Could you check a few things on this model? Use its own coordinates, in mm. A direction names the side the tool comes from. Give positions to 0.01 mm unless a question says otherwise; leave off trailing zeros. Order: outer loops, then holes, each group sorted by start corner. A loop starts at its lowest first (then second) coordinate and runs counter-clockwise, first axis right, second up. Notation, with made-up numbers: (-37, 53) -> (-17, 53) arc R14 ccw to (-17, 70) -> close; hole circle Ø4 at (85.25, 76.25). An arc over 180 degrees is marked (long way). Write each question's results on one line, items separated by ' | '.
```python
from build123d import *
from build123d.topology import SkipClean

# Parameters (mm, degrees)
SKETCH1_R           = 1.6
BOSS_EXTRUDE1_DEPTH = 20
SKETCH3_R           = 2.6
BOSS_EXTRUDE2_DEPTH = 15


with BuildPart() as part:
    # Sketch1 → Boss-Extrude1 (new body)
    with BuildSketch(Plane(origin=(0, 0, 0), x_dir=(1, 0, 0), z_dir=(0, 1, 0))):
        with BuildLine():
            Line((165, -10), (165, 0))
            Line((165, 0), (84, 0))
            Line((84, 0), (84, -4))
            Line((84, -4), (149, -4))
            ThreePointArc((149, -4), (153.242640687, -5.757359313), (155, -10))
            ThreePointArc((155, -10), (160, -15), (165, -10))
        make_face()
        with Locations(Location((160, -10, 0), (0, 0, 270))):
            Circle(SKETCH1_R, mode=Mode.SUBTRACT)
    extrude(amount=BOSS_EXTRUDE1_DEPTH)


with BuildPart() as body_2:
    # Sketch3 → Boss-Extrude2 (new, through all)
    with BuildSketch(Plane.XY):
        with BuildLine():
            Line((122, 0), (165, 0))
            Line((165, 0), (165, 9))
            Line((165, 9), (153.284271247, 9))
            ThreePointArc((153.284271247, 9), (149.457436924, 9.761204675), (146.213203436, 11.928932188))
            Line((146.213203436, 11.928932188), (141.071067812, 17.071067812))
            ThreePointArc((141.071067812, 17.071067812), (137.826834324, 19.238795325), (134, 20))
            Line((134, 20), (84, 20))
            Line((84, 20), (84, 12.6))
            ThreePointArc((84, 12.6), (85.838477631, 11.838477631), (86.6, 10))
            ThreePointArc((86.6, 10), (85.838477631, 8.161522369), (84, 7.4))
            Line((84, 7.4), (84, 0))
            Line((84, 0), (114, 0))
            ThreePointArc((114, 0), (118, 4), (122, 0))
        make_face()
        with Locations((134, 10)):
            Circle(SKETCH3_R, mode=Mode.SUBTRACT)
    extrude(amount=BOSS_EXTRUDE2_DEPTH)

    # Intersect1: read off the stored shape, not the designer's step
    # Intersect1: intersect part
    add(part.part, mode=Mode.INTERSECT)

    # Mirror1: body 2 across face


with BuildPart() as body_2_1:
    with SkipClean():  # the faces are left unmerged after this step: merging them gives an invalid solid
        add(body_2.part)
        add(body_2.part.mirror(Plane(origin=(84, 16.3, 2), x_dir=(0, 0, 1), z_dir=(-1, 0, 0))))


solid = body_2_1.part
```
Q1. Thinking about a two-plate mould opening in X: for faces 1 (the flat face through (85, 5, 4)), 2 (the flat face through (15, 0, 4)), 3 (the cylindrical face through (149.51, 9.74, 2.21)), 4 (the cylindrical face through (8.97, 4.44, 8.73)), which applies, +X half, -X half, draft (parallel to the pull), parting line (faces both ways), or undercut?
Here are the results:
face 1: undercut | face 2: draft | face 3: +X half | face 4: undercut
Q2. I'm going to push flat-ended pins straight in: pin 1 Ø4 at (x, z) = (8, 10) entering from +Y; pin 2 Ø1 at (x, z) = (72, 2.5) entering from -Y; pin 3 Ø1 at (x, y) = (116.5, 16.5) entering from +Z; pin 4 Ø5 at (y, z) = (16.5, 5) entering from -X. Where does each tip first touch, or does it pass through?
Here are the results:
pin 1: stops at y = 9 | pin 2: stops at y = 0 | pin 3: stops at z = 4 | pin 4: stops at x = 24.07
Q3. Suppose I cut it at C-C on z = 13.5. Please give me the cut outline in (x, y), and give its area (3 significant figures).
Here are the results:
outline: (4.43, 0) -> (11.57, 0) -> (11.57, 9) -> (4.43, 9) -> close; (156.43, 0) -> (163.57, 0) -> (163.57, 9) -> (156.43, 9) -> close | area: 129 mm²
Q4. I need wall thicknesses on line 1 along X through (y, z) = (6.75, 10); line 2 along Z through (x, y) = (8, 3.75); line 3 along X through (y, z) = (2, 9.25). Which ranges of each line are inside material? Lowest first, please.
Here are the results:
line 1: x = 3 to 6.4, 9.6 to 13, 155 to 158.4, 161.6 to 165 | line 2: z = 0 to 8.4, 11.6 to 15 | line 3: x = 3 to 6.59, 9.41 to 13.05, 154.95 to 158.59, 161.41 to 165
Q5. Suppose I cut it at D-D on x = 44.5. Please give me the cut outline in (y, z).
Here are the results:
outline: (0, 0) -> (20, 0) -> (20, 4) -> (0, 4) -> close
Q6. Suppose I cut it at A-A on x = 160. Please give me the cut outline in (y, z).
Here are the results:
outline: (0, 0) -> (9, 0) -> (9, 8.4) -> (0, 8.4) -> close; (0, 11.6) -> (9, 11.6) -> (9, 15) -> (0, 15) -> close
Q7. Suppose I cut it at B-B on z = 2.5. Please give me the cut outline in (x, y), and give its area (3 significant figures).
Here are the results:
outline: (3, 0) -> (46, 0) arc R4 cw to (54, 0) -> (114, 0) arc R4 cw to (122, 0) -> (165, 0) -> (165, 9) -> (153.28, 9) arc R10 cw to (146.21, 11.93) -> (141.07, 17.07) arc R10 ccw to (134, 20) -> (34, 20) arc R10 ccw to (26.93, 17.07) -> (21.79, 11.93) arc R10 cw to (14.72, 9) -> (3, 9) -> close; hole circle Ø5.2 at (34, 10); hole circle Ø5.2 at (84, 10); hole circle Ø5.2 at (134, 10) | area: 2,660 mm²
Q8. For faces 5 (the flat face through (9, 9, 6)), 6 (the flat face through (159, 9, 6)), 7 (the cylindrical face through (153.196, 4.912, 5.711)), 8 (the cylindrical face through (118, 4, 2)), which set-ups out of +Z, -Z, +X, -X, +Y, -Y let a thin tool reach every point of the face, with its end or its side?
Here are the results:
face 5: +Z, -Z, -X, +Y | face 6: +Z, -Z, +X, +Y | face 7: +Z, +Y, -Y | face 8: +Z, -Z, -Y
